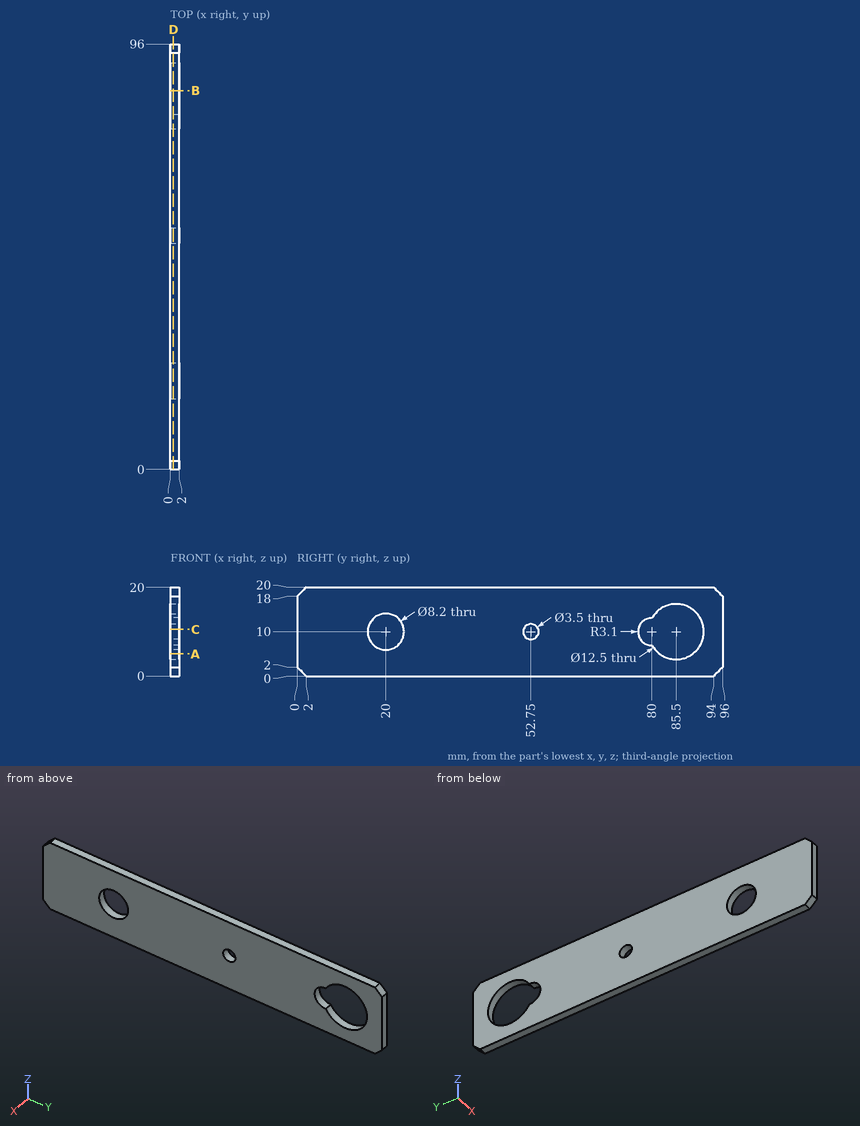
Drawing for the job (mm, zero at the part's lowest x, y, z). Round coordinates to 2 decimals unless told otherwise and drop trailing zeros. Loops run counter-clockwise (first coordinate to the right, second up) from the corner with the lowest first, then second, coordinate; pieces in that order, holes last. Notation, with made-up numbers: (35.25, -22.5) -> (40.25, -22.5) arc R15 ccw to (40.25, 6.5) -> close; hole circle Ø9 at (27, 42). An arc over 180 degrees is marked (long way). Use one line per item in the form item = value. Start each with the question number.
Item 1: Drill centre lines: line 1 along Y through (x, z) = (0.6, 10); line 2 along Y through (x, z) = (0.85, 7.25); line 3 along Y through (x, z) = (1.7, 8). Where is each one in solid material? Low to high.
Item 2: Band-saw the part on A-A (z = 5). List the corners of the cut face in (x, y), plus the area to 3 significant figures.
Item 3: Drop a flat-ended pin along its axis: pin 1 Ø2 at (y, z) = (52.75, 10) entering from -X. Give the stop position or say it passes through.
Item 4: Band-saw the part on D-D (x = 0.7). List the corners of the cut face in (y, z).
Item 5: Band-saw the part on B-B (y = 85.5). List the corners of the cut face in (x, z), plus the area to 3 significant figures.
Item 6: Band-saw the part on C-C (z = 10.5). List the corners of the cut face in (x, y).
Data:
q1.line_1 = 0 to 15.9, 24.1 to 51, 54.5 to 76.9, 91.75 to 96
q1.line_2 = 0 to 16.96, 23.04 to 78.57, 91.11 to 96
q1.line_3 = 0 to 16.42, 23.58 to 77.63, 91.42 to 96
q2.outline = (0, 0) -> (2, 0) -> (2, 81.75) -> (0, 81.75) -> close; (0, 89.25) -> (2, 89.25) -> (2, 96) -> (0, 96) -> close
q2.area = 177 mm^2
q3.pin_1 = through
q4.outline = (0, 2) -> (2, 0) -> (94, 0) -> (96, 2) -> (96, 18) -> (94, 20) -> (2, 20) -> (0, 18) -> close; hole circle Ø8.2 at (20, 10); hole circle Ø3.5 at (52.75, 10); hole (80.07, 6.9) arc R6.25 ccw (long way) to (80.07, 13.1) arc R3.1 ccw (long way) to start
q5.outline = (0, 0) -> (2, 0) -> (2, 3.75) -> (0, 3.75) -> close; (0, 16.25) -> (2, 16.25) -> (2, 20) -> (0, 20) -> close
q5.area = 15.0 mm^2
q6.outline = (0, 0) -> (2, 0) -> (2, 15.93) -> (0, 15.93) -> close; (0, 24.07) -> (2, 24.07) -> (2, 51.07) -> (0, 51.07) -> close; (0, 54.43) -> (2, 54.43) -> (2, 76.94) -> (0, 76.94) -> close; (0, 91.73) -> (2, 91.73) -> (2, 96) -> (0, 96) -> close
